Verification items for this drawing (mm, ordinates from the low corner). A direction names the side the tool comes from. Round coordinates to 2 decimals unless told otherwise and drop trailing zeros. Loops run counter-clockwise (first coordinate to the right, second up) from the corner with the lowest first, then second, coordinate; pieces in that order, holes last. Notation, with made-up numbers: M 9,37 L 19,37 A15 cw 19,46 Z; hole C -33.75,89 d1. An arc over 180 degrees is marked long. Write item = value, one per line. Start each with the question number.
(1) Scan lines: L1, parallel to Z at x = 19, y = 8.75; L2, parallel to X at y = 9.25, z = 6; L3, parallel to X at y = 9.75, z = 12 (1 decimal). Record each from-to range of solid material in increasing order. Write a range as from..to.
(2) Cross-section at C-C on z = 14. Record the boundary of the cut face in (x, y), plus the area to 3 significant figures.
(3) Go/stop test with flat-tipped pins: P1, Ø6, axis at y = 15.5, z = 5.5, coming from the +X side; P2, Ø3, axis at x = 9, z = 6, coming from the +Y side; P3, Ø5, axis at x = 16.5, z = 5.5, coming from the -Y side. Record where each tip stops, or that it passes through.
(4) Cross-section at B-B on x = 7.75. Record the boundary of the cut face in (y, z) (1 decimal), plus the area to 3 significant figures.
(5) Cross-section at D-D on x = 18.5. Record the boundary of the cut face in (y, z), plus the area to 3 significant figures.
(6) Set-up check for the marked faces 1, 2, 3, 4 and 5: record each of +Z, -Z, +X, -X, +Y, -Y from which the full face is reachable in a straight line by a thin tool's end or side.
(7) Cross-section at A-A on x = 2.25. Record the boundary of the cut face in (y, z).
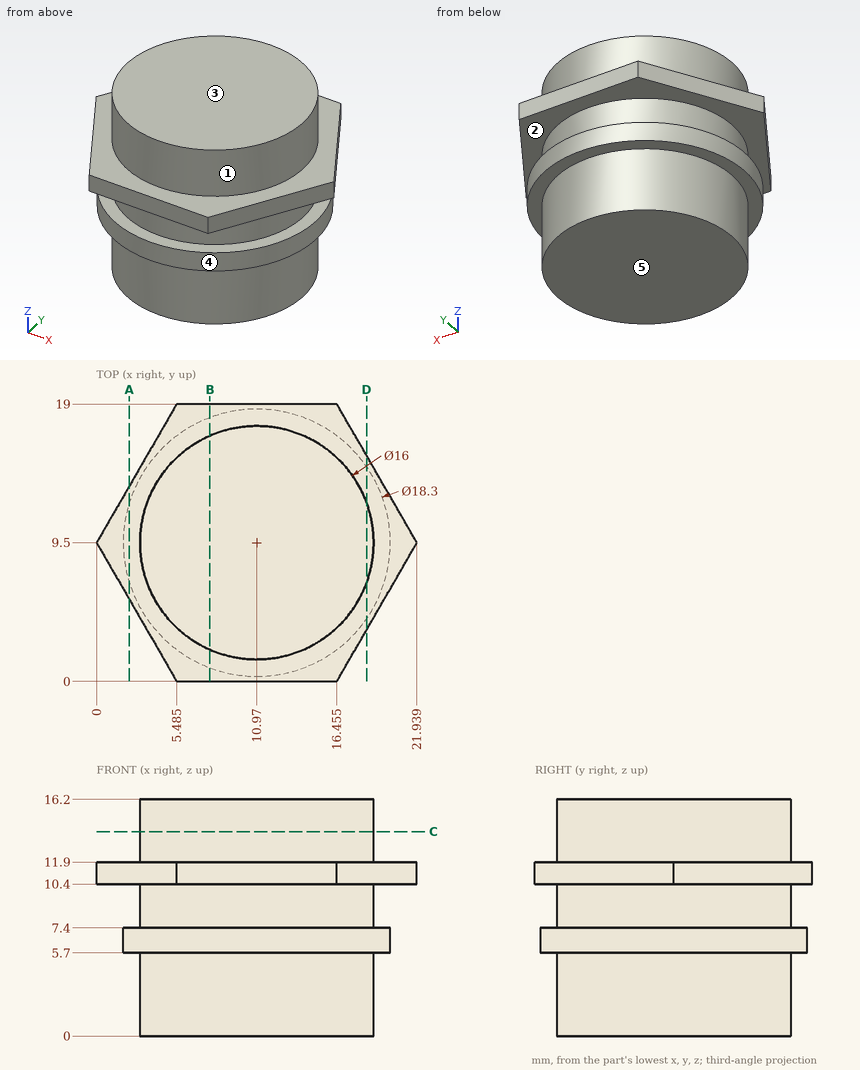
Result:
q1.L1 = 5.7..7.4, 10.4..11.9
q1.L2 = 1.82..20.12
q1.L3 = 3..19
q2.outline = C 10.97,9.5 d16
q2.area = 201 mm^2
q3.P1 = 19.61
q3.P2 = 18.64
q3.P3 = 0.87
q4.outline = M 0,10.4 L 2.2,10.4 L 2.2,7.4 L 0.9,7.4 L 0.9,5.7 L 2.2,5.7 L 2.2,0 L 16.8,0 L 16.8,5.7 L 18.1,5.7 L 18.1,7.4 L 16.8,7.4 L 16.8,10.4 L 19,10.4 L 19,11.9 L 16.8,11.9 L 16.8,16.2 L 2.2,16.2 L 2.2,11.9 L 0,11.9 Z
q4.area = 248 mm^2
q5.outline = M 3.54,10.4 L 6.8,10.4 L 6.8,7.4 L 4.3,7.4 L 4.3,5.7 L 6.8,5.7 L 6.8,0 L 12.2,0 L 12.2,5.7 L 14.7,5.7 L 14.7,7.4 L 12.2,7.4 L 12.2,10.4 L 15.46,10.4 L 15.46,11.9 L 12.2,11.9 L 12.2,16.2 L 6.8,16.2 L 6.8,11.9 L 3.54,11.9 Z
q5.area = 106 mm^2
q6.face_1 = +Z
q6.face_2 = none
q6.face_3 = +Z, +X, -X, +Y, -Y
q6.face_4 = -Z
q6.face_5 = -Z, +X, -X, +Y, -Y
q7.outline = M 5.6,10.4 L 13.4,10.4 L 13.4,11.9 L 5.6,11.9 Z; M 6.73,5.7 L 12.27,5.7 L 12.27,7.4 L 6.73,7.4 Z
